Could you check a few things on this model? Use its own coordinates, in mm. Give positions to 0.01 mm unless a question says otherwise; leave off trailing zeros. Loops run counter-clockwise (first coordinate to the right, second up) from the corner with the lowest first, then second, coordinate; pieces in that order, holes last. Notation, with made-up numbers: M 10,41 L 42,41 A14 cw 42,52 Z; hole C 8.5,64 d8. An arc over 180 degrees is marked long. Use a Markdown table: item, result. Add a question column.
1) If I drill on line 1 along Z through (x, y) = (0, 17); line 2 along X through (y, z) = (64, 657); line 3 along X through (y, z) = (-0.5, 601), over which ranges is the centre line in solid material (lowest first)? Write a range as [from, to].
2) Will these pins go through, and if not, where does the flat tip stop? pin 1 Ø4 at (x, z) = (32.5, 344) entering from -Y; pin 2 Ø4 at (y, z) = (-8, 553.5) entering from +X; pin 3 Ø10 at (x, z) = (-25.5, 353) entering from +Y.
3) We'd pull the mould along Y, two halves only. Please class faces 1 (the cylindrical face through (-9.764, 74.362, 345.1)), 2 (the flat face through (-1, 1, 0)): +Y half, -Y half, draft (parallel to the pull), parting line (faces both ways), or undercut.
4) Suppose I cut it at B-B on z = 417.5. List the corners of the cut face in (x, y) for me.
5) Suppose I cut it at A-A on y = -45. List the corners of the cut face in (x, z) for me, and give its area (3 significant figures).
6) Suppose I cut it at C-C on x = 40.5. List the corners of the cut face in (y, z) for me, and give its area (3 significant figures).
7) Suppose I cut it at D-D on y = 52.5. List the corners of the cut face in (x, z) for me, and give its area (3 significant figures).
```python
from build123d import *

# Parameters (mm, degrees)
SCHIZZO1_R                    = 75
ESTRUSIONE_ESTRUSIONE1_DEPTH  = 700
TAGLIO_ESTRUSIONE1_DEPTH      = 708.990112925
TAGLIO_ESTRUSIONE1_DEPTH_BACK = 708.990112925
SCHIZZO2_R                    = 5
TAGLIO_ESTRUSIONE2_DEPTH      = 708.990113045
TAGLIO_ESTRUSIONE2_DEPTH_BACK = 708.990113045
SCHIZZO3_R                    = 5


with BuildPart() as part:
    # Schizzo1 → Estrusione-Estrusione1 (new body)
    with BuildSketch(Plane.XY):
        Circle(SCHIZZO1_R)
    extrude(amount=ESTRUSIONE_ESTRUSIONE1_DEPTH)

    # Schizzo2 → Taglio-Estrusione1 (cut, two sides: drawn at the far end of the back side and taken through both)
    with BuildSketch(Plane(origin=(0, 0, 0), x_dir=(1, 0, 0), z_dir=(0, 1, 0)).offset(-TAGLIO_ESTRUSIONE1_DEPTH_BACK)):
        with Locations(Location((0, -43.632162592, 0), (0, 0, 270))):
            Circle(SCHIZZO2_R)
    extrude(amount=TAGLIO_ESTRUSIONE1_DEPTH + TAGLIO_ESTRUSIONE1_DEPTH_BACK, mode=Mode.SUBTRACT)

    # Schizzo3 → Taglio-Estrusione2 (cut, two sides: drawn at the far end of the back side and taken through both)
    with BuildSketch(Plane(origin=(0, 0, 0), x_dir=(1, 0, 0), z_dir=(0, 1, 0)).offset(-TAGLIO_ESTRUSIONE2_DEPTH_BACK)):
        with Locations(Location((0, -659.26265162, 0), (0, 0, 270))):
            Circle(SCHIZZO3_R)
    extrude(amount=TAGLIO_ESTRUSIONE2_DEPTH + TAGLIO_ESTRUSIONE2_DEPTH_BACK, mode=Mode.SUBTRACT)


solid = part.part
```
Answer block:
| question | item | result |
|---|---|---|
| 1 | line 1 | z = [0, 38.63], [48.63, 654.26], [664.26, 700] |
| 1 | line 2 | x = [-39.1, -4.46], [4.46, 39.1] |
| 1 | line 3 | x = [-75, 75] |
| 2 | pin 1 | stops at y = -68.52 |
| 2 | pin 2 | stops at x = 74.76 |
| 2 | pin 3 | stops at y = 72.14 |
| 3 | face 1 | parting line |
| 3 | face 2 | draft |
| 4 | outline | C 0,0 d150 |
| 5 | outline | M -60,0 L 60,0 L 60,700 L -60,700 Z; hole C 0,43.63 d10; hole C 0,659.26 d10 |
| 5 | area | 83,800 mm^2 |
| 6 | outline | M -63.12,0 L 63.12,0 L 63.12,700 L -63.12,700 Z |
| 6 | area | 88,400 mm^2 |
| 7 | outline | M -53.56,0 L 53.56,0 L 53.56,700 L -53.56,700 Z; hole C 0,43.63 d10; hole C 0,659.26 d10 |
| 7 | area | 74,800 mm^2 |
